from build123d import *

# Parameters (mm, degrees)
EXTRUDE_1_DEPTH     = 18
FILLET_1_R          = 2
SKETCH_2_R          = 4.4
SKETCH_2_R_2        = 2.75
CUT_EXTRUDE_1_DEPTH = 10
SKETCH_3_R          = 4.4
CUT_EXTRUDE_2_DEPTH = 10


with BuildPart() as part:
    # 草图1 → 凸台-拉伸1 (new body)
    with BuildSketch(Plane.XY):
        Polygon((0, 0), (-48.5, 0), (-48.5, 48), (-50.5, 48), (-50.5, -2), (0, -2), align=None)
    extrude(amount=EXTRUDE_1_DEPTH)

    # 圆角1
    fillet_1_edges = [part.edges().sort_by_distance(p)[0] for p in [
        (-48.5, 0, 9),
    ]]
    fillet(fillet_1_edges, radius=FILLET_1_R)

    # 草图2 → 切除-拉伸1 (cut)
    with BuildSketch(Plane(origin=(-48.5, 0, 0), x_dir=(0, 0, -1), z_dir=(1, 0, 0))):
        with BuildLine():
            Line((-9, 48), (-18, 48))
            Line((-18, 48), (-18, 39))
            ThreePointArc((-18, 39), (-15.363961031, 45.363961031), (-9, 48))
        make_face()
        with Locations((-9, 21)):
            Circle(SKETCH_2_R)
        with Locations((-9, 37)):
            Circle(SKETCH_2_R_2)
        with BuildLine():
            Line((0, 48), (-9, 48))
            ThreePointArc((-9, 48), (-2.636038969, 45.363961031), (0, 39))
            Line((0, 39), (0, 48))
        make_face()
    extrude(amount=-CUT_EXTRUDE_1_DEPTH, mode=Mode.SUBTRACT)

    # 草图3 → 切除-拉伸2 (cut)
    with BuildSketch(Plane(origin=(0, 0, 0), x_dir=(1, 0, 0), z_dir=(0, 1, 0))):
        with BuildLine():
            Line((0, -9), (0, 0))
            Line((0, 0), (-9, 0))
            ThreePointArc((-9, 0), (-2.636038969, -2.636038969), (0, -9))
        make_face()
        with Locations(Location((-34, -9, 0), (0, 0, 270))):
            Circle(SKETCH_3_R)
        with Locations(Location((-11, -9, 0), (0, 0, 270))):
            Circle(SKETCH_3_R)
        with BuildLine():
            Line((0, -18), (0, -9))
            ThreePointArc((0, -9), (-2.636038969, -15.363961031), (-9, -18))
            Line((-9, -18), (0, -18))
        make_face()
    extrude(amount=-CUT_EXTRUDE_2_DEPTH, mode=Mode.SUBTRACT)


solid = part.part
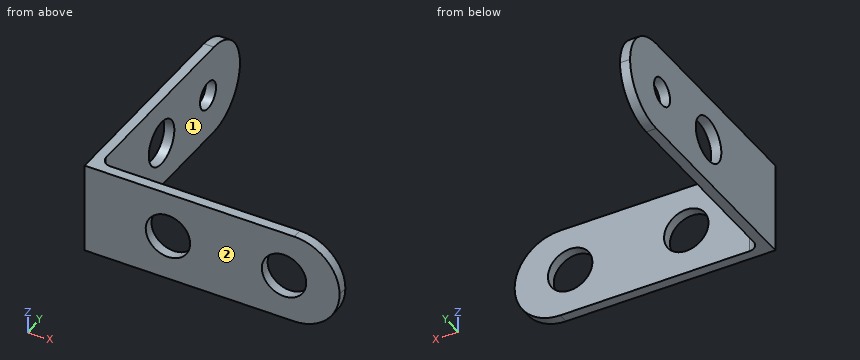
CAD build for the part. Positions are in the model's coordinates, mm. Face numbers are marked on the shaded views. A direction names the side the tool comes from. Round coordinates to 2 decimals unless told otherwise and drop trailing zeros. Write each loop counter-clockwise with the first axis right and the second up, starting at its lowest first coordinate (ties: lowest second). Pieces come first, ordered by that corner, then holes. Notation, with made-up numbers: M 81,43.25 L 104,43.25 A3 ccw 104,48.25 Z; hole C -4.5,14 d7. An arc over 180 degrees is marked long. Use a Markdown table: item, result. Add a question column.
1. Slice it at D-D on z = 7.25. Give the cut face in (x, y), then the cut area to 3 significant figures.
2. Drill centre lines: probe 1 along Y at (x, z) = (-49.95, 9); probe 2 along X at (y, z) = (-1.25, 9); probe 3 along Y at (x, z) = (-43, 15.75). Where is each one in solid material? Low to high.
3. Slice it at C-C on z = 11. Give the cut face in (x, y), then the cut area to 3 significant figures.
4. 3-axis set-ups, long thin cutter, end or side, ignore diameter. For the marked faces 1 and 2: which of +Z, -Z, +X, -X, +Y, -Y reach the whole face in a straight line?
5. Flat gauge pins, fed straight in: P1, Ø1, axis at x = -15.5, z = 4, coming from the +Y side; P2, Ø1.5, axis at y = 27.5, z = 11.5, coming from the +X side; P3, Ø5, axis at y = 37, z = 9, coming from the +X side. Where does each tip first touch, or does it go through?
6. Slice it at B-B on y = 21. Give the cut face in (x, z).
7. Slice it at A-A on x = -34. Give the cut face in (y, z).
Reply:
| question | item | result |
|---|---|---|
| 1 | outline | M -50.5,-2 L -38.04,-2 L -38.04,0 L -46.5,0 A2 cw -48.5,2 L -48.5,16.96 L -50.5,16.96 Z; M -50.5,25.04 L -48.5,25.04 L -48.5,34.88 L -50.5,34.88 Z; M -50.5,39.12 L -48.5,39.12 L -48.5,47.83 L -50.5,47.83 Z; M -29.96,-2 L -15.04,-2 L -15.04,0 L -29.96,0 Z; M -6.96,-2 L -0.17,-2 L -0.17,0 L -6.96,0 Z |
| 1 | area | 140 mm^2 |
| 2 | probe 1 | y = -2 to 16.6, 25.4 to 34.25, 39.75 to 48 |
| 2 | probe 2 | x = -50.5 to -38.4, -29.6 to -15.4, -6.6 to 0 |
| 2 | probe 3 | y = -2 to 0 |
| 3 | outline | M -50.5,-2 L -37.92,-2 L -37.92,0 L -46.5,0 A2 cw -48.5,2 L -48.5,17.08 L -50.5,17.08 Z; M -50.5,24.92 L -48.5,24.92 L -48.5,35.11 L -50.5,35.11 Z; M -50.5,38.89 L -48.5,38.89 L -48.5,47.77 L -50.5,47.77 Z; M -30.08,-2 L -14.92,-2 L -14.92,0 L -30.08,0 Z; M -7.08,-2 L -0.23,-2 L -0.23,0 L -7.08,0 Z |
| 3 | area | 142 mm^2 |
| 4 | face 1 | +Z, -Z, +X, +Y |
| 4 | face 2 | +Z, -Z, +X, -X, -Y |
| 5 | P1 | stops at y = 0 |
| 5 | P2 | stops at x = -48.5 |
| 5 | P3 | passes through |
| 6 | outline | M -50.5,0 L -48.5,0 L -48.5,4.6 L -50.5,4.6 Z; M -50.5,13.4 L -48.5,13.4 L -48.5,18 L -50.5,18 Z |
| 7 | outline | M -2,0 L 0,0 L 0,4.6 L -2,4.6 Z; M -2,13.4 L 0,13.4 L 0,18 L -2,18 Z |
